from build123d import *

# Parameters (mm, degrees)
BOSS_EXTRUDE1_DEPTH            = 4
SLOT_ALIGNER_DEPTH             = 2
ALIGNER_DEPTH                  = 2
DEBURS_SIZE                    = 0.2
CBORE_FOR_M3_SHCS1_D           = 3.4
CBORE_FOR_M3_SHCS1_CBORE_D     = 6.5
CBORE_FOR_M3_SHCS1_CBORE_DEPTH = 3
CHAMFER1_SIZE                  = 0.2


with BuildPart() as part:
    # Sketch1 → Boss-Extrude1 (new body)
    with BuildSketch(Plane.XY):
        Polygon((-21.3, -6), (21.3, -6), (21.5, -5.8), (21.5, 5.8), (21.3, 6), (14.2, 6), (14, 5.8), (14, -4), (-14, -4), (-14, 5.8), (-14.2, 6), (-21.3, 6), (-21.5, 5.8), (-21.5, -5.8), align=None)
    extrude(amount=-BOSS_EXTRUDE1_DEPTH)

    # Sketch3 → Slot Aligner (add)
    with BuildSketch(Plane.XY):
        Polygon((15.95, 3.552468642), (14, 4.917873342), (14, 0.082126658), (15.95, 1.447531358), align=None)
    slot_aligner = extrude(amount=SLOT_ALIGNER_DEPTH)

    # Mirror3: Slot Aligner across plane
    add(slot_aligner.mirror(Plane(origin=(0, 0, 0), x_dir=(0, 0, 1), z_dir=(1, 0, 0))))

    # Sketch4 → Aligner (add)
    with BuildSketch(Plane(origin=(0, 0, 0), x_dir=(-1, 0, 0), z_dir=(0, 0, -1))):
        Polygon((-19.8, 1.958578644), (-21.4, 3.558578644), (-21.5, 3.658578644), (-21.5, -1.658578644), (-21.4, -1.558578644), (-19.8, 0.041421356), align=None)
    aligner = extrude(amount=-ALIGNER_DEPTH)

    # Aligners: Aligner across plane
    add(aligner.mirror(Plane(origin=(0, 0, 0), x_dir=(0, 0, 1), z_dir=(1, 0, 0))))

    # Deburs
    deburs_edges = [part.edges().sort_by_distance(p)[0] for p in [
        (-14.1, 5.9, -4),
        (-17.75, 6, -4),
        (-21.4, 5.9, -4),
        (-21.5, 0, -4),
        (-21.4, -5.9, -4),
        (0, -6, -4),
        (21.4, -5.9, -4),
        (21.5, 0, -4),
        (21.4, 5.9, -4),
        (15.95, 2.5, 2),
        (14.975, 4.235170992, 2),
        (14.975, 0.764829008, 2),
        (17.75, 6, -4),
        (0, -4, -4),
        (14.1, 5.9, -4),
        (14, 0.9, -4),
        (-15.95, 2.5, 2),
        (-14.975, 0.764829008, 2),
        (-14.975, 4.235170992, 2),
        (19.8, 1, 2),
        (20.65, -0.808578644, 2),
        (20.65, 2.808578644, 2),
        (-19.8, 1, 2),
        (-20.65, 2.808578644, 2),
        (-20.65, -0.808578644, 2),
        (-14, 0.9, -4),
    ]]
    chamfer(deburs_edges, length=DEBURS_SIZE)

    # CBORE for M3 SHCS1 (through all)
    with Locations(Plane(origin=(0, 0, -4), x_dir=(-1, 0, 0), z_dir=(0, 0, -1))):
        with Locations((-17.75, -2.25), (17.75, -2.25)):
            CounterBoreHole(CBORE_FOR_M3_SHCS1_D / 2, CBORE_FOR_M3_SHCS1_CBORE_D / 2, CBORE_FOR_M3_SHCS1_CBORE_DEPTH)

    # Chamfer1
    chamfer1_edges = [part.edges().sort_by_distance(p)[0] for p in [
        (-19.45, -2.25, 0),
        (-14.5, -2.25, -4),
        (-19.45, -2.25, -1),
        (16.05, -2.25, 0),
        (21, -2.25, -4),
        (16.05, -2.25, -1),
    ]]
    chamfer(chamfer1_edges, length=CHAMFER1_SIZE)


solid = part.part
Geometry check sheet. Reference: the model listing, model coordinates, mm. A direction names the side the tool comes from. Give positions to 0.01 mm unless a question says otherwise; leave off trailing zeros. Loops run counter-clockwise (first coordinate to the right, second up) from the corner with the lowest first, then second, coordinate; pieces in that order, holes last. Notation, with made-up numbers: (32, -27) -> (70, -27) arc R28 cw to (70, 11) -> close; hole circle Ø8 at (72, 60.5). An arc over 180 degrees is marked (long way). Answer in a Markdown table with one row per item. Add a question column.
1) Gauge pin test, flat ends, axial feed: P1, Ø4, axis at x = -17.75, y = -2.25, coming from the -Z side; P2, Ø4, axis at x = -10.5, y = -3.5, coming from the +Z side; P3, Ø2, axis at x = -18.5, y = -2.5, coming from the -Z side. Record the tip position at first contact, or that the pin passes through.
2) Draft check along Y on faces 5 (the face through (-14, 1, -2)), 6 (the face through (20.997, -2.107, -2.42)), 7 (the face through (0, -6, -2)). Enter one of: pulls with the +Y half, pulls with the -Y half, needs draft (parallel to the pull), parting line crosses it, or undercut.
3) Cross-section at B-B on x = -17.75. Record the boundary of the cut face in (y, z).
4) Cross-section at A-A on z = -2.5. Record the boundary of the cut face in (x, y).
5) Cross-section at D-D on x = -11. Record the boundary of the cut face in (y, z).
6) Material ranges on probe 1 along Y at (x, z) = (-17.75, -0.7); probe 2 along X at (y, z) = (5.5, -2.5); probe 3 along Y at (x, z) = (-17.75, -1.85), recorded low to high. Write a range as from..to.
7) Cross-section at C-C on y = -2.25. State how many separate pieces and enclosed holes the cut face has, and give its area (3 significant figures).
8) Set-up check for faces 1 (the face through (-14.961, 0.755, 0.887)), 2 (the face through (15.95, 2, 1)), 3 (the face through (21, 1, 2)), 4 (the face through (-20.64, 2.8, 0.89)): record each of +Z, -Z, +X, -X, +Y, -Y from which the full face is reachable in a straight line by a thin tool's end or side.
Outcome:
| question | item | result |
|---|---|---|
| 1 | P1 | stops at z = -1 |
| 1 | P2 | stops at z = 0 |
| 1 | P3 | stops at z = -0.89 |
| 2 | face 5 | needs draft |
| 2 | face 6 | undercut |
| 2 | face 7 | pulls with the -Y half |
| 3 | outline | (-6, -3.8) -> (-5.8, -4) -> (-5.7, -4) -> (-5.5, -3.8) -> (-5.5, -1) -> (-4.15, -1) -> (-3.95, -0.8) -> (-3.95, -0.2) -> (-4.15, 0) -> (-6, 0) -> close; (-0.55, -0.8) -> (-0.35, -1) -> (1, -1) -> (1, -3.8) -> (1.2, -4) -> (5.8, -4) -> (6, -3.8) -> (6, 0) -> (-0.35, 0) -> (-0.55, -0.2) -> close |
| 4 | outline | (-21.5, -5.8) -> (-21.3, -6) -> (21.3, -6) -> (21.5, -5.8) -> (21.5, 5.8) -> (21.3, 6) -> (14.2, 6) -> (14, 5.8) -> (14, -4) -> (-14, -4) -> (-14, 5.8) -> (-14.2, 6) -> (-21.3, 6) -> (-21.5, 5.8) -> close; hole circle Ø6.5 at (-17.75, -2.25); hole circle Ø6.5 at (17.75, -2.25) |
| 5 | outline | (-6, -3.8) -> (-5.8, -4) -> (-4.2, -4) -> (-4, -3.8) -> (-4, 0) -> (-6, 0) -> close |
| 6 | probe 1 | y = -6..-3.95, -0.55..6 |
| 6 | probe 2 | x = -21.5..-14, 14..21.5 |
| 6 | probe 3 | y = -6..-5.5, 1..6 |
| 7 | separate pieces | 4 |
| 7 | enclosed holes | 0 |
| 7 | area | 13.9 mm^2 |
| 8 | face 1 | +Z, -Y |
| 8 | face 2 | +Z, +Y, -Y |
| 8 | face 3 | +Z, +X, -X, +Y, -Y |
| 8 | face 4 | +Z, +Y |
